Geometry check sheet. Reference: the model listing, model coordinates, mm. Face numbers are marked on the shaded views. A direction names the side the tool comes from. Give positions to 0.01 mm unless a question says otherwise; leave off trailing zeros. Loops run counter-clockwise (first coordinate to the right, second up) from the corner with the lowest first, then second, coordinate; pieces in that order, holes last. Notation, with made-up numbers: (0.5, -0.5) -> (39.5, -0.5) arc R34 cw to (39.5, 33.5) -> close; hole circle Ø11 at (45, -13.75). An arc over 180 degrees is marked (long way). One line per question, with ' | ' between items.
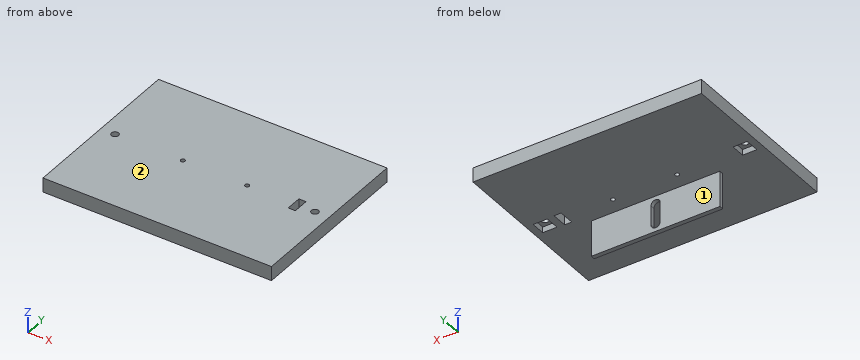
from build123d import *

# Parameters (mm, degrees)
SKETCH1_W           = 160
SKETCH1_H           = 120
BOSS_EXTRUDE1_DEPTH = 10
SKETCH2_R           = 1.5
SKETCH2_R_2         = 2.5
SKETCH2_W           = 5
SKETCH2_H           = 11
CUT_EXTRUDE2_DEPTH  = 101.498756211
SKETCH3_W           = 10
SKETCH3_H           = 10
CUT_EXTRUDE3_DEPTH  = 4
SKETCH4_W           = 90
SKETCH4_H           = 3
BOSS_EXTRUDE3_DEPTH = 25.05
CUT_EXTRUDE5_DEPTH  = 112.819061434


with BuildPart() as part:
    # Sketch1 → Boss-Extrude1 (new body)
    with BuildSketch(Plane.XY):
        Rectangle(SKETCH1_W, SKETCH1_H)
    extrude(amount=BOSS_EXTRUDE1_DEPTH)

    # Sketch2 → Cut-Extrude2 (cut, through all)
    with BuildSketch(Plane(origin=(0, 0, 0), x_dir=(-1, 0, 0), z_dir=(0, 0, -1))):
        with Locations((-22.5, 0)):
            Circle(SKETCH2_R)
        with Locations((22.5, 0)):
            Circle(SKETCH2_R)
        with Locations((70, 0)):
            Circle(SKETCH2_R_2)
        with Locations((-70, 0)):
            Circle(SKETCH2_R_2)
        with Locations((-57.5, 0)):
            Rectangle(SKETCH2_W, SKETCH2_H)
    extrude(amount=-CUT_EXTRUDE2_DEPTH, mode=Mode.SUBTRACT)

    # Sketch3 → Cut-Extrude3 (cut)
    with BuildSketch(Plane(origin=(0, 0, 0), x_dir=(-1, 0, 0), z_dir=(0, 0, -1))):
        with Locations((-70, 0)):
            Rectangle(SKETCH3_W, SKETCH3_H)
        with Locations((70, 0)):
            Rectangle(SKETCH3_W, SKETCH3_H)
    extrude(amount=-CUT_EXTRUDE3_DEPTH, mode=Mode.SUBTRACT)

    # Sketch4 → Boss-Extrude3 (add)
    with BuildSketch(Plane(origin=(0, 0, 0), x_dir=(-1, 0, 0), z_dir=(0, 0, -1))):
        with Locations((0, -12.5)):
            Rectangle(SKETCH4_W, SKETCH4_H)
    extrude(amount=BOSS_EXTRUDE3_DEPTH)

    # Sketch5 → Cut-Extrude5 (cut, through all)
    with BuildSketch(Plane.XZ.offset(14)):
        with BuildLine():
            Line((3.2, -19.325), (3.2, -5.725))
            ThreePointArc((3.2, -5.725), (0, -2.525), (-3.2, -5.725))
            Line((-3.2, -5.725), (-3.2, -19.325))
            ThreePointArc((-3.2, -19.325), (0, -22.525), (3.2, -19.325))
        make_face()
    extrude(amount=-CUT_EXTRUDE5_DEPTH, mode=Mode.SUBTRACT)


solid = part.part
Item 1: Scan lines: probe 1 along Y at (x, z) = (22.5, 4); probe 2 along Z at (x, y) = (68, 9); probe 3 along Y at (x, z) = (70, 7.1). Record each from-to range of solid material in increasing order.
Result:
probe 1: -60 to -1.5, 1.5 to 60 | probe 2: 0 to 10 | probe 3: -60 to -2.5, 2.5 to 60
Item 2: Depth check by flat-ended pin: pin 1 Ø3.5 at (y, z) = (-13, -18.5) entering from +X; pin 2 Ø3 at (y, z) = (24.5, -0.5) entering from -X; pin 3 Ø1.5 at (x, y) = (-38.5, -19.5) entering from -Z; pin 4 Ø1.5 at (y, z) = (-12.5, -13) entering from -X. Enter the tip coordinate at first touch or a pass-through.
Result:
pin 1: x = 45 | pin 2: x = -80 | pin 3: z = 0 | pin 4: x = -45
Item 3: Sectioned sample at D-D (x = 1.5). Record the cut outline in (y, z).
Result:
outline: (-60, 0) -> (-14, 0) -> (-14, -2.9) -> (-11, -2.9) -> (-11, 0) -> (60, 0) -> (60, 10) -> (-60, 10) -> close; (-14, -25.05) -> (-11, -25.05) -> (-11, -22.15) -> (-14, -22.15) -> close
Item 4: Sectioned sample at B-B (x = 36). Record the cut outline in (y, z), plus the area to 3 significant figures.
Result:
outline: (-60, 0) -> (-14, 0) -> (-14, -25.05) -> (-11, -25.05) -> (-11, 0) -> (60, 0) -> (60, 10) -> (-60, 10) -> close | area: 1,280 mm2
Item 5: Set-up check for the marked faces 1 and 2: record each of +Z, -Z, +X, -X, +Y, -Y from which the full face is reachable in a straight line by a thin tool's end or side.
Result:
face 1: -Z, +X, -X, +Y | face 2: +Z, +X, -X, +Y, -Y
Item 6: Sectioned sample at C-C (y = 39.5). Record the cut outline in (x, z).
Result:
outline: (-80, 0) -> (80, 0) -> (80, 10) -> (-80, 10) -> close
Item 7: Sectioned sample at A-A (x = -70). Record the cut outline in (y, z).
Result:
outline: (-60, 0) -> (-5, 0) -> (-5, 4) -> (-2.5, 4) -> (-2.5, 10) -> (-60, 10) -> close; (2.5, 4) -> (5, 4) -> (5, 0) -> (60, 0) -> (60, 10) -> (2.5, 10) -> close
